from build123d import *

# Parameters (mm, degrees)
F0_W     = 9.525
F0_H     = 76.2
F1_DEPTH = 9.525
F2_W     = 8.001
F2_H     = 5.08
F3_DEPTH = 25.4
F4_R     = 39.221374
F5_DEPTH = 25.4
F7_DEPTH = 25.4


with BuildPart() as f1:
    # F0 (on Top) → F1 (new body)
    with BuildSketch(Plane.XY):
        with Locations((4.7625, 38.1)):
            Rectangle(F0_W, F0_H)
    extrude(amount=F1_DEPTH)

    # F2 (on face) → F3 (cut)
    with BuildSketch(Plane.XY.offset(9.525)):
        Polygon((1.524, 0), (1.524, -3.864633), (13.939685, -4.220638), (13.939685, 5.08), (9.525, 5.08), (9.525, 0), align=None)
        with Locations((5.5245, 2.54)):
            Rectangle(F2_W, F2_H)
    extrude(amount=-F3_DEPTH, mode=Mode.SUBTRACT)

    # F4 (on face) → F5 (cut)
    with BuildSketch(Plane.YZ.offset(9.525)):
        with Locations((2.740548, 48.620269)):
            Circle(F4_R)
    extrude(amount=-F5_DEPTH, mode=Mode.SUBTRACT)

    # F6 (on face) → F7 (cut)
    with BuildSketch(Plane.YZ.offset(9.525)):
        Polygon((2.305606, -2.034316), (0, 9.494759), (0, 0), align=None)
    extrude(amount=-F7_DEPTH, mode=Mode.SUBTRACT)


solid = f1.part
Check sheet for the modelled part. Datum: model origin and axes. Units: mm. A direction names the side the tool comes from. Coordinates: 2 decimals unless noted, no trailing zeros. Write each loop counter-clockwise with the first axis right and the second up, starting at its lowest first coordinate (ties: lowest second). Pieces come first, ordered by that corner, then holes.
Item 1: Depth check by flat-ended pin: pin 1 Ø1 at (x, z) = (3.5, 4.5) entering from -Y; pin 2 Ø4 at (y, z) = (2, 3) entering from +X. Enter the tip coordinate at first touch or a pass-through.
Numbers:
pin 1: stops at y = 5.08
pin 2: stops at x = 1.52
Item 2: Access from +Z, -Z, +X, -X, +Y, -Y to the whole of each face (thin tool, end or side, straight path). Record for faces 1 (the face through (6, 5.08, 5)), 2 (the face through (0, 38, 5)).
Numbers:
face 1: +Z, -Z, +X, -Y
face 2: +Z, -Z, -X, +Y, -Y
Item 3: Cross-section at B-B on z = 1.75. Record the boundary of the cut face in (x, y) (3 decimals).
Numbers:
outline: (0, 1.549) - (1.524, 1.549) - (1.524, 5.08) - (9.525, 5.08) - (9.525, 76.2) - (0, 76.2) - close
Item 4: Scan lines: probe 1 along Z at (x, y) = (2.25, 5.5); probe 2 along Y at (x, z) = (7.25, 8); probe 3 along X at (y, z) = (4, 5). Record each from-to range of solid material in increasing order.
Numbers:
probe 1: z = 0 to 9.5
probe 2: y = 5.08 to 76.2
probe 3: x = 0 to 1.52
Item 5: Cross-section at A-A on x = 6.5. Record the boundary of the cut face in (y, z) (3 decimals), then the cut area to 3 significant figures.
Numbers:
outline: (5.08, 0) - (76.2, 0) - (76.2, 9.525) - (5.883, 9.525) arc R39.221 cw to (5.08, 9.469) - close
area: 677 mm2
Item 6: Cross-section at C-C on z = 4.75. Record the boundary of the cut face in (x, y) (3 decimals), then the cut area to 3 significant figures.
Numbers:
outline: (0, 0.949) - (1.524, 0.949) - (1.524, 5.08) - (9.525, 5.08) - (9.525, 76.2) - (0, 76.2) - close
area: 684 mm2
